Part model, mm, in its own coordinate system. A direction names the side the tool comes from. Give positions to 0.01 mm unless a question says otherwise; leave off trailing zeros. Answer in a Markdown table with one row per item. Add a question column.
1. Which spindle directions (+Z, -Z, +X, -X, +Y, -Y) get a long thin tool onto all of the face, cutting with end or side? Do faces 5 (the flat face through (0, -1, 5.906)), 6 (the conical face through (-5.798, 1.218, 1.099)). Say none if no direction does.
2. Pull direction X, two halves, no side cores. Call faces 1 (the flat face through (-3.3, 4.3, -2.032)), 2 (the flat face through (-3.5, 0.1, 4.318)), 3 (the flat face through (-4.62, -5.63, 1.88)), 4 (the flat face through (1.25, 5.63, 1.88)): released by +X, released by -X, zero draft, split by the parting line, or undercut.
3. Drop flat-ended pins along their axis: pin 1 Ø1 at (y, z) = (3, 0) entering from +X; pin 2 Ø6 at (x, y) = (-2.5, 0) entering from -Z; pin 3 Ø1 at (y, z) = (5, 3) entering from -X. Give the stop position or say it passes through.
4. Probe line 1 along X through (y, z) = (1.5, 3.5); line 2 along Z through (x, y) = (-1.25, 3.5); line 3 along X through (y, z) = (2.5, 3). List the from-to ranges inside material, lowest first.
Autodesk Inventor part; units mm, degrees
ref_plane "Work Plane3" through (-1.6844, 0, -2.032) normal (0, 0, 1) x (0.9993818, 0.0351571, 0)
ref_plane "YZ Plane" through (0, 0, 0) normal (1, 0, 0) x (0, 1, 0)
ref_plane "XZ Plane" through (0, 0, 0) normal (0, 1, 0) x (-1, 0, 0)
ref_plane "Work Plane3" through (-1.6844, 0, -2.032) normal (0, 0, 1) x (0.9993818, 0.0351571, 0)
sketch "Sketch6" plane through (-1.6844, 0, -2.032) normal (0, 0, 1) x (0.9993818, 0.0351571, 0)
  circle A0 centre (0, 0) radius 6.35
  line L0 (0, 7.3323) -> (6.35, 3.6662)
  line L1 (6.35, 3.6662) -> (6.35, -3.6662)
  line L2 (6.35, -3.6662) -> (0, -7.3323)
  line L3 (0, -7.3323) -> (-6.35, -3.6662)
  line L4 (-6.35, -3.6662) -> (-6.35, 3.6662)
  line L5 (-6.35, 3.6662) -> (0, 7.3323)
  point P0 (1.6833, -0.0592)
  point P1 (0, 7.8524)
  dimension "d5" = 12.7
extrude "Extrusion2" add sketch "Sketch6" along normal blind 7.9375
sketch "Sketch7" plane through (-1.6844, 0, -2.032) normal (0, 0, -1) x (-0.9993818, -0.0351571, 0)
  circle A0 centre (-0.0028, 0.0799) radius 4.3656
  point P0 (-1.6833, -0.0592)
extrude "Extrusion3" cut sketch "Sketch7" against normal blind 6.35 draft -1.783
sketch "Sketch8" plane through (-1.6844, 0, 5.9055) normal (0, 0, 1) x (0.9993818, 0.0351571, 0)
  circle A0 centre (0.0028, 0.0799) radius 1.651
  point P0 (1.6833, -0.0592)
extrude "Extrusion4" cut sketch "Sketch8" against normal through all
thread "Thread1"
ref_plane "Work Plane4" through (-1.9422, 7.3278, -2.032) normal (0.9993818, 0.0351571, 0) x (0, 0, 1)
sketch "Sketch9" plane through (-1.9422, 7.3278, -2.032) normal (0.9993818, 0.0351571, 0) x (0, 0, 1)
  line L0 (7.9375, 13.5217) -> (7.593, 14.6647)
  line L1 (7.593, 14.6647) -> (7.9375, 13.5217)
  line L2 (7.593, 14.6647) -> (7.9375, 14.6647)
  line L3 (7.9375, 14.6647) -> (7.9375, 13.5217)
  line L4 (9.525, 7.2525) -> (-1.5875, 7.2525)
  point P0 (2.032, 7.3916)
  dimension "d13" = 1.143
revolve "Revolution2" cut sketch "Sketch9" angle 360 about axis through (-1.6872, 0.0798, 5.9055) along (0, 0, -1)
ref_plane "Work Plane5" through (-1.6872, 0.0798, 1.9367) normal (0, 0, 1) x (1, 0, 0)
mirror "Mirror1" about plane through (-1.6872, 0.0798, 1.9367) normal (0, 0, 1) of "Revolution2"
properties part number "Pneumatics_VIAIR_Fitting_01"
Values:
| question | item | result |
|---|---|---|
| 1 | face 5 | +Z, +X, -X, +Y, -Y |
| 1 | face 6 | -Z |
| 2 | face 1 | zero draft |
| 2 | face 2 | undercut |
| 2 | face 3 | released by -X |
| 2 | face 4 | released by +X |
| 3 | pin 1 | stops at x = 4.58 |
| 3 | pin 2 | stops at z = 4.32 |
| 3 | pin 3 | stops at x = -6.47 |
| 4 | line 1 | x = -8.09 to -5.63, 2.26 to 4.62 |
| 4 | line 2 | z = 4.32 to 5.91 |
| 4 | line 3 | x = -8.13 to -5.13, 1.76 to 4.58 |
